For this review, take the finished solid that the model builds, in its own axes (mm). Coordinates: 2 decimals unless noted, no trailing zeros. Order: outer loops, then holes, each group sorted by start corner. A loop starts at its lowest first (then second) coordinate and runs counter-clockwise, first axis right, second up. Notation, with made-up numbers: (85, 3.25) -> (93, 3.25) arc R27 ccw to (93, 40.25) -> close; hole circle Ø5 at (-17, -24). An arc over 180 degrees is marked (long way). Answer as a JSON object with one key per item and string values. Group by question number.
1) Add section D-D, the plane z = -72. Write out the cut boundary in (x, y), then the cut area to 3 significant figures.
2) For pin 1 (0.9 mm diameter, centred on y = 2, z = -187, fed in from -X), flat-tipped, find the tip position at first contact; note if it passes through.
3) Wall thickness on L1, parallel to X at y = 1, z = -42.5; L2, parallel to Z at x = 31.5, y = 0.1; L3, parallel to Z at x = 85.5, y = 1.85: over which ranges is each line inside the solid? List them lowest first.
4) Add section A-A, the plane x = 79.5. Write out the cut boundary in (y, z), then the cut area to 3 significant figures.
5) Add section B-B, the plane z = -133. Write out the cut boundary in (x, y), then the cut area to 3 significant figures.
6) Add section C-C, the plane y = 2.1. Count the separate pieces of the cut face and the enclosed holes in it, then the cut area to 3 significant figures.
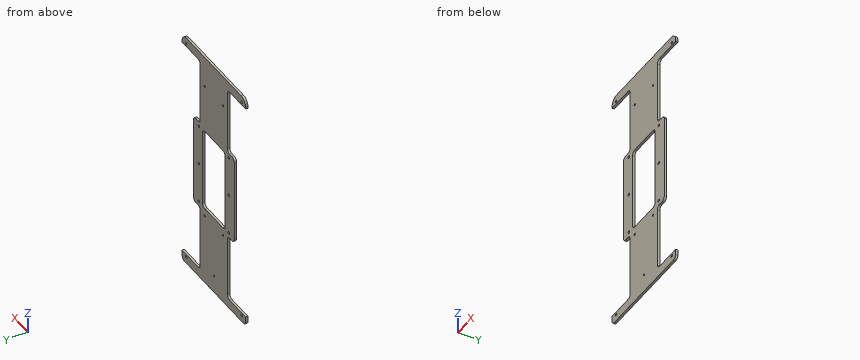
from build123d import *

# Parameters (mm, degrees)
BOSS_EXTRUDE1_DEPTH = 3
FILLET1_R           = 10
FILLET2_R           = 5
SKETCH2_R           = 1.65
CUT_EXTRUDE1_DEPTH  = 359.481519747
SKETCH3_R           = 1.65
CUT_EXTRUDE2_DEPTH  = 359.481519747
SKETCH4_R           = 1.65
CUT_EXTRUDE3_DEPTH  = 359.481519747
FILLET3_R           = 5
SKETCH5_R           = 1.35
CUT_EXTRUDE4_DEPTH  = 10
SKETCH6_W           = 50
SKETCH6_H           = 113
CUT_EXTRUDE5_DEPTH  = 10
FILLET4_R           = 5


with BuildPart() as part:
    # Sketch1 → Boss-Extrude1 (new body)
    with BuildSketch(Plane(origin=(0, 0, 0), x_dir=(1, 0, 0), z_dir=(0, 1, 0))):
        Polygon((0, 0), (140, 0), (140, 12.5), (100, 12.5), (100, 103.5), (115, 103.5), (115, 226.5), (100, 226.5), (100, 317.5), (140, 317.5), (140, 330), (0, 330), (0, 317.5), (40, 317.5), (40, 226.5), (25, 226.5), (25, 103.5), (40, 103.5), (40, 12.5), (0, 12.5), align=None)
    extrude(amount=BOSS_EXTRUDE1_DEPTH)

    # Fillet1
    fillet1_edges = [part.edges().sort_by_distance(p)[0] for p in [
        (140, 1.5, 0),
        (0, 1.5, 0),
    ]]
    fillet(fillet1_edges, radius=FILLET1_R)

    # Fillet2
    fillet2_edges = [part.edges().sort_by_distance(p)[0] for p in [
        (25, 1.5, -103.5),
        (25, 1.5, -226.5),
        (0, 1.5, -330),
        (140, 1.5, -330),
        (115, 1.5, -226.5),
        (115, 1.5, -103.5),
    ]]
    fillet(fillet2_edges, radius=FILLET2_R)

    # Sketch2 → Cut-Extrude1 (cut, through all)
    with BuildSketch(Plane(origin=(0, 3, 0), x_dir=(1, 0, 0), z_dir=(0, 1, 0))):
        with Locations(Location((37, 220, 0), (0, 0, 270))):
            Circle(SKETCH2_R)
        with Locations(Location((37, 165, 0), (0, 0, 270))):
            Circle(SKETCH2_R)
        with Locations(Location((37, 110, 0), (0, 0, 270))):
            Circle(SKETCH2_R)
        with Locations(Location((103, 110, 0), (0, 0, 90))):
            Circle(SKETCH2_R)
        with Locations(Location((103, 165, 0), (0, 0, 90))):
            Circle(SKETCH2_R)
        with Locations(Location((103, 220, 0), (0, 0, 90))):
            Circle(SKETCH2_R)
    extrude(amount=-CUT_EXTRUDE1_DEPTH, mode=Mode.SUBTRACT)

    # Sketch3 → Cut-Extrude2 (cut, through all)
    with BuildSketch(Plane(origin=(0, 3, 0), x_dir=(1, 0, 0), z_dir=(0, 1, 0))):
        with Locations(Location((8.75, 8.75, 0), (0, 0, 270))):
            Circle(SKETCH3_R)
        with Locations(Location((131.25, 8.75, 0), (0, 0, 90))):
            Circle(SKETCH3_R)
    extrude(amount=-CUT_EXTRUDE2_DEPTH, mode=Mode.SUBTRACT)

    # Sketch4 → Cut-Extrude3 (cut, through all)
    with BuildSketch(Plane(origin=(0, 3, 0), x_dir=(1, 0, 0), z_dir=(0, 1, 0))):
        with Locations(Location((8.75, 321.25, 0), (0, 0, 270))):
            Circle(SKETCH4_R)
        with Locations(Location((131.25, 321.25, 0), (0, 0, 90))):
            Circle(SKETCH4_R)
    extrude(amount=-CUT_EXTRUDE3_DEPTH, mode=Mode.SUBTRACT)

    # Fillet3
    fillet3_edges = [part.edges().sort_by_distance(p)[0] for p in [
        (40, 1.5, -12.5),
        (40, 1.5, -103.5),
        (40, 1.5, -226.5),
        (40, 1.5, -317.5),
        (100, 1.5, -317.5),
        (100, 1.5, -226.5),
        (100, 1.5, -103.5),
        (100, 1.5, -12.5),
    ]]
    fillet(fillet3_edges, radius=FILLET3_R)

    # Sketch5 → Cut-Extrude4 (cut)
    with BuildSketch(Plane(origin=(0, 3, 0), x_dir=(1, 0, 0), z_dir=(0, 1, 0))):
        with Locations(Location((50, 42.5, 0), (0, 0, 270))):
            Circle(SKETCH5_R)
        with Locations(Location((90, 42.5, 0), (0, 0, 270))):
            Circle(SKETCH5_R)
        with Locations(Location((50, 232.5, 0), (0, 0, 270))):
            Circle(SKETCH5_R)
        with Locations(Location((90, 232.5, 0), (0, 0, 270))):
            Circle(SKETCH5_R)
        with Locations(Location((70, 306.15, 0), (0, 0, 270))):
            Circle(SKETCH5_R)
    extrude(amount=-CUT_EXTRUDE4_DEPTH, mode=Mode.SUBTRACT)

    # Sketch6 → Cut-Extrude5 (cut)
    with BuildSketch(Plane(origin=(0, 3, 0), x_dir=(1, 0, 0), z_dir=(0, 1, 0))):
        with Locations((70, 165)):
            Rectangle(SKETCH6_W, SKETCH6_H)
    extrude(amount=-CUT_EXTRUDE5_DEPTH, mode=Mode.SUBTRACT)

    # Fillet4
    fillet4_edges = [part.edges().sort_by_distance(p)[0] for p in [
        (45, 1.5, -108.5),
        (45, 1.5, -221.5),
        (95, 1.5, -221.5),
        (95, 1.5, -108.5),
    ]]
    fillet(fillet4_edges, radius=FILLET4_R)


solid = part.part
Output values:
{
 "1": {"outline": "(40, 0) -> (100, 0) -> (100, 3) -> (40, 3) -> close", "area": "180 mm²"},
 "2": {"pin 1": "stops at x = 25"},
 "3": {"L1": "x = 40 to 48.65, 51.35 to 88.65, 91.35 to 100", "L2": "z = -330 to -317.5, -226.5 to -103.5, -12.5 to 0", "L3": "z = -330 to -221.5, -108.5 to 0"},
 "4": {"outline": "(0, -330) -> (3, -330) -> (3, -221.5) -> (0, -221.5) -> close; (0, -108.5) -> (3, -108.5) -> (3, 0) -> (0, 0) -> close", "area": "651 mm²"},
 "5": {"outline": "(25, 0) -> (45, 0) -> (45, 3) -> (25, 3) -> close; (95, 0) -> (115, 0) -> (115, 3) -> (95, 3) -> close", "area": "120 mm²"},
 "6": {"separate pieces": "1", "enclosed holes": "16", "area": "19,700 mm²"}
}
